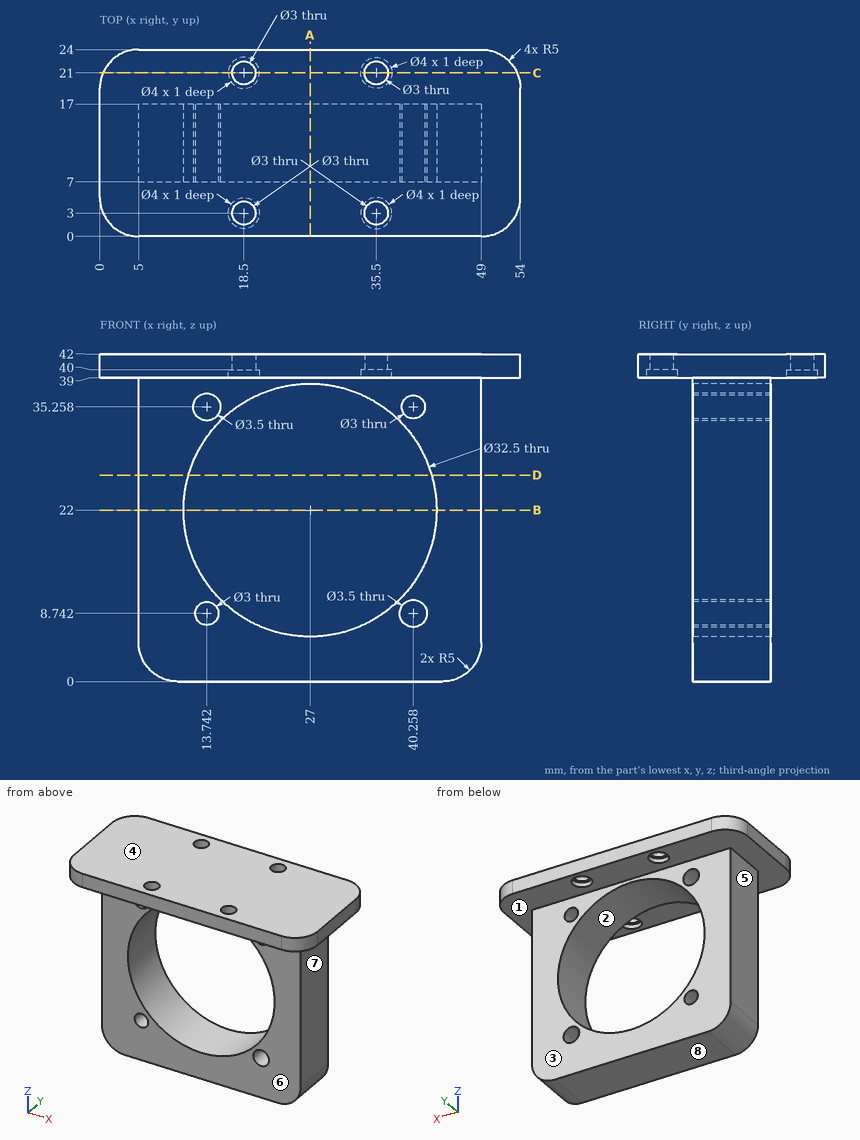
Study the drawing (mm; zero at the part's minimum x, y, z) and answer. A direction names the side the tool comes from. Give positions to 0.01 mm unless a question says otherwise; leave off trailing zeros. Order: outer loops, then holes, each group sorted by start corner. A loop starts at its lowest first (then second) coordinate and runs counter-clockwise, first axis right, second up. Notation, with made-up numbers: M 65.25,17.5 L 111.25,17.5 A15 ccw 111.25,21.5 Z; hole C 40,18 d4. An arc over 180 degrees is marked long. Put each result on its own line as item: value. Start each with the question number.
Item 1: The part is cut by section A-A, the plane x = 27. Determine the outline of the cut face in (y, z).
Item 2: The part is cut by section D-D, the plane z = 26.5. Determine the outline of the cut face in (x, y) (1 decimal).
Item 3: The part is cut by section C-C, the plane y = 21. Determine the outline of the cut face in (x, z).
Item 4: Find the intervals of material crossed by line 1 along Y through (x, z) = (18.5, 40.5); line 2 along X through (y, z) = (11, 35.5) (1 decimal); line 3 along Z through (x, y) = (13.5, 16.5) (1 decimal), in increasing order.
Item 5: For a pull along Z with two mould halves and no side action, classify the marked faces 1, 2 and 3 as +Z half, -Z half, draft (parallel to the pull), parting line (faces both ways), or undercut.
Item 6: Flat-ended cylindrical pins translate along their axes: P1, Ø3.5, axis at x = 18.5, y = 3, coming from the -Z side; P2, Ø1, axis at y = 8.5, z = 9.5, coming from the -X side; P3, Ø5, axis at x = 38.5, z = 10, coming from the +Y side; P4, Ø10, axis at x = 31, y = 21, coming from the -Z side. Find the tip coordinate at first contact, or state that the pin passes through.
Item 7: The part is cut by section B-B, the plane z = 22. Determine the outline of the cut face in (x, y), and give its area (3 significant figures).
Item 8: Which of the six approach directions +Z, -Z, +X, -X, +Y, -Y give full straight-line access (tool end or side, diameter ignored) to the marked faces 4, 5, 6, 7 and 8?
Answer key:
1. outline: M 0,39 L 7,39 L 7,38.25 L 17,38.25 L 17,39 L 24,39 L 24,42 L 0,42 Z; M 7,0 L 17,0 L 17,5.75 L 7,5.75 Z
2. outline: M 5,7 L 11.4,7 L 11.4,17 L 5,17 Z; M 42.6,7 L 49,7 L 49,17 L 42.6,17 Z
3. outline: M 0.42,39 L 16.5,39 L 16.5,40 L 17,40 L 17,42 L 0.42,42 Z; M 20,40 L 20.5,40 L 20.5,39 L 33.5,39 L 33.5,40 L 34,40 L 34,42 L 20,42 Z; M 37,40 L 37.5,40 L 37.5,39 L 53.58,39 L 53.58,42 L 37,42 Z
4. line 1: y = 0 to 1.5, 4.5 to 19.5, 22.5 to 24
4. line 2: x = 5 to 12, 15.5 to 18, 36 to 38.8, 41.7 to 49
4. line 3: z = 0 to 7.3, 10.2 to 13, 31 to 33.5, 37 to 42
5. face 1: -Z half
5. face 2: undercut
5. face 3: draft
6. P1: stops at z = 40
6. P2: stops at x = 5
6. P3: stops at y = 17
6. P4: stops at z = 0
7. outline: M 5,7 L 10.75,7 L 10.75,17 L 5,17 Z; M 43.25,7 L 49,7 L 49,17 L 43.25,17 Z
7. area: 115 mm²
8. face 4: +Z, +X, -X, +Y, -Y
8. face 5: -Z, -X, +Y, -Y
8. face 6: -Z, +X, -X, -Y
8. face 7: -Z, +X, +Y, -Y
8. face 8: -Z, +X, -X, +Y, -Y
